Read the model definition and answer for the solid it produces. Units are mm, in the model's axes. A direction names the side the tool comes from. Round coordinates to 2 decimals unless told otherwise and drop trailing zeros. Order: outer loops, then holes, each group sorted by start corner. A loop starts at its lowest first (then second) coordinate and runs counter-clockwise, first axis right, second up. Notation, with made-up numbers: (16.5, -4) - (63.5, -4) arc R25 ccw to (63.5, 28) - close; hole circle Ø11 at (-16.5, 40.25). An arc over 180 degrees is marked (long way). Answer as a JSON object with one key per item and string values. Group by question number.
Q1. Given pin 1 Ø2 at (x, z) = (-0.5, -0.5) entering from +Y; pin 2 Ø4 at (x, y) = (1, 4) entering from +Z; pin 3 Ø1 at (x, y) = (3.5, 18.5) entering from +Z; pin 4 Ø4 at (y, z) = (17.5, 4) entering from +X, each flat-ended and moving along its own axis, determine where each tip first touches the part or whether it passes through.
Q2. A cutting plane is placed at D-D on x = 1.75. Determine the outline of the cut face in (y, z), and give its area (3 significant figures).
Q3. A cutting plane is placed at C-C on y = 15.75. Determine the outline of the cut face in (x, z).
Q4. Consider line 1 (X direction, y = 21.2, z = 0); line 2 (Z direction, x = 1.5, y = 10.5); line 3 (Z direction, x = 0.25, y = 17.5). Determine where each line is inside the solid, lowest interval first.
Q5. A cutting plane is placed at B-B on z = 0. Determine the outline of the cut face in (x, y), and give its area (3 significant figures).
Q6. The mould has two halves that part along X. Classify faces 4 (the flat face through (-0.1, 0, 3.3)), 5 (the flat face through (-1, 13, -1)), 6 (the cylindrical face through (0, 12, -5)): pulls with the +X half, pulls with the -X half, needs draft (parallel to the pull), parting line crosses it, or undercut.
Q7. A tool of negligible diameter and unlimited length cuts with its end or side. For faces 1 (the cylindrical face through (-0.9, 6.59, 2.86)), 2 (the cylindrical face through (2, 21, 0)), 3 (the flat face through (-0.1, 24, -2.2)), from which of +Z, -Z, +X, -X, +Y, -Y can it reach the whole face along a straight path? Write none if from no direction.
Q8. A cutting plane is placed at A-A on x = 0. Determine the outline of the cut face in (y, z).
```python
from build123d import *

# Parameters (mm, degrees)
SKETCH3_R           = 3
SKETCH3_R_2         = 1
BOSS_EXTRUDE1_DEPTH = 5


with BuildPart() as part:
    # Sketch2 → Revolve1 (revolve)
    with BuildSketch(Plane.XY, mode=Mode.PRIVATE) as revolve1_sk:
        Polygon((3, 0), (3, 18), (2, 18), (2, 24), (5, 24), (5, 0), align=None)
    revolve(revolve1_sk.sketch.rotate(Axis((0, 10.839741494, 0), (0, -1, 0)), 90), axis=Axis((0, 10.839741494, 0), (0, -1, 0)))

    # Sketch3 → Boss-Extrude1 (add)
    with BuildSketch(Plane.XZ.offset(-18)):
        with Locations(Location((0, 0, 0), (0, 0, 90))):
            Circle(SKETCH3_R)
        with Locations(Location((0, 0, 0), (0, 0, 270))):
            Circle(SKETCH3_R_2, mode=Mode.SUBTRACT)
    extrude(amount=BOSS_EXTRUDE1_DEPTH)


solid = part.part
```
Result set:
{
 "1": {"pin 1": "stops at y = 18", "pin 2": "stops at z = 5", "pin 3": "stops at z = 4", "pin 4": "stops at x = 4.58"},
 "2": {"outline": "(0, -4.68) - (24, -4.68) - (24, -0.97) - (18, -0.97) - (18, 0.97) - (24, 0.97) - (24, 4.68) - (0, 4.68) - (0, 2.44) - (13, 2.44) - (13, -2.44) - (0, -2.44) - close", "area": "150 mm²"},
 "3": {"outline": "circle Ø10 at (0, 0); hole circle Ø2 at (0, 0)"},
 "4": {"line 1": "x = -5 to -2, 2 to 5", "line 2": "z = -4.77 to -2.6, 2.6 to 4.77", "line 3": "z = -4.99 to -0.97, 0.97 to 4.99"},
 "5": {"outline": "(-5, 0) - (-3, 0) - (-3, 13) - (-1, 13) - (-1, 18) - (-2, 18) - (-2, 24) - (-5, 24) - close; (1, 13) - (3, 13) - (3, 0) - (5, 0) - (5, 24) - (2, 24) - (2, 18) - (1, 18) - close", "area": "128 mm²"},
 "6": {"face 4": "needs draft", "face 5": "undercut", "face 6": "parting line crosses it"},
 "7": {"face 1": "-Y", "face 2": "+Y", "face 3": "+Z, -Z, +X, -X, +Y"},
 "8": {"outline": "(0, -5) - (24, -5) - (24, -2) - (18, -2) - (18, -1) - (13, -1) - (13, -3) - (0, -3) - close; (0, 3) - (13, 3) - (13, 1) - (18, 1) - (18, 2) - (24, 2) - (24, 5) - (0, 5) - close"}
}
